Can you work these out from the model? Positions are in its coordinate system, mm. A direction names the side the tool comes from. Round coordinates to 2 decimals unless told otherwise and drop trailing zeros. Write each loop counter-clockwise with the first axis right and the second up, starting at its lowest first coordinate (ties: lowest second). Pieces come first, ordered by that corner, then holes. Notation, with made-up numbers: (35, 60.5) -> (77, 60.5) arc R26 cw to (77, 74.5) -> close; hole circle Ø6 at (54.5, -40). An arc over 180 degrees is marked (long way). Write item = value, one per line. Start each with the question number.
1) Thinking about a two-plate mould opening in X: for faces 1 (the face through (-56.53, 26.78, 0.99)), 2 (the face through (-45, -47.4, 16)), 3 (the face through (15, -42.9, 1)), which applies, +X half, -X half, draft (parallel to the pull), parting line (faces both ways), or undercut?
2) If I drill on line 1 (Y direction, x = 27.5, z = 15.75); line 2 (X direction, y = -44.5, z = 6.25); line 3 (Z direction, x = -13.5, y = 5.5), over which ranges is the centre line in solid material (lowest first)?
3) Imagine slicing it at B-B, the plane z = 11.5. Please give me the cut outline in (x, y).
4) Imagine slicing it at D-D, the plane z = 4. Please give me the cut outline in (x, y), then the cut area to 3 significant figures.
5) For faces 4 (the face through (-27.068, 3.734, 0.986)), 5 (the face through (-34.01, -42.94, 0.99)), 6 (the face through (26.01, -43.743, 8.902)), which set-ups out of +Z, -Z, +X, -X, +Y, -Y let a thin tool reach every point of the face, with its end or its side?
6) I'm going to push flat-ended pins straight in: pin 1 (5.5 mm diameter, centred on x = 20.53, y = 20.83, fed in from +Z); pin 2 (1.4 mm diameter, centred on x = 28, y = -47, fed in from +Z); pin 3 (0.6 mm diameter, centred on x = -9, z = 1.5, fed in from -Y). Where does each tip first touch, or does it pass through?
7) Imagine slicing it at A-A, the plane y = 9. Please give me the cut outline in (x, z).
8) Imagine slicing it at C-C, the plane x = -22.5. Please give me the cut outline in (y, z), then the cut area to 3 significant figures.
from build123d import *

# Parameters (mm, degrees)
SKETCH1_R           = 13
SKETCH1_R_2         = 3
BOSS_EXTRUDE1_DEPTH = 2
SKETCH2_R           = 3.3
BOSS_EXTRUDE2_DEPTH = 14
SKETCH3_R           = 1.4
CUT_EXTRUDE1_DEPTH  = 10


with BuildPart() as part:
    # Sketch1 → Boss-Extrude1 (new body)
    with BuildSketch(Plane.XY):
        with BuildLine():
            Line((30.587032828, 29.429180606), (-49.522529265, 29.429180606))
            ThreePointArc((-49.522529265, 29.429180606), (-56.615313692, 26.706515756), (-60.064461355, 19.937182317))
            Line((-60.064461355, 19.937182317), (-65.933159759, -35.899753171))
            ThreePointArc((-65.933159759, -35.899753171), (-55.634580371, -52.232565016), (-37.345276376, -46.042020648))
            ThreePointArc((-37.345276376, -46.042020648), (-33.948223744, -42.907324122), (-29.467749897, -41.770819394))
            Line((-29.467749897, -41.770819394), (10.53225346, -41.770819394))
            ThreePointArc((10.53225346, -41.770819394), (15.012727307, -42.907324122), (18.409779939, -46.042020648))
            ThreePointArc((18.409779939, -46.042020648), (36.699083934, -52.232565016), (46.997663323, -35.899753171))
            Line((46.997663323, -35.899753171), (41.128964919, 19.937182317))
            ThreePointArc((41.128964919, 19.937182317), (37.679817255, 26.706515756), (30.587032828, 29.429180606))
        make_face()
        with Locations((-39.467748218, -0.170819394)):
            Circle(SKETCH1_R, mode=Mode.SUBTRACT)
        with Locations(Location((20.532251782, -0.170819394, 0), (0, 0, 180))):
            Circle(SKETCH1_R, mode=Mode.SUBTRACT)
        with Locations((-39.467748218, 20.829180606)):
            Circle(SKETCH1_R_2, mode=Mode.SUBTRACT)
        with Locations(Location((20.532251782, 20.829180606, 0), (0, 0, 180))):
            Circle(SKETCH1_R_2, mode=Mode.SUBTRACT)
    extrude(amount=BOSS_EXTRUDE1_DEPTH)

    # Sketch2 → Boss-Extrude2 (add)
    with BuildSketch(Plane.XY.offset(2)):
        with Locations((-46.467748218, -46.670819394)):
            Circle(SKETCH2_R)
        with Locations(Location((27.532251782, -46.670819394, 0), (0, 0, 180))):
            Circle(SKETCH2_R)
    extrude(amount=BOSS_EXTRUDE2_DEPTH)

    # Sketch3 → Cut-Extrude1 (cut)
    with BuildSketch(Plane.XY.offset(16)):
        with Locations((-46.467748218, -46.670819394)):
            Circle(SKETCH3_R)
        with Locations(Location((27.532251782, -46.670819394, 0), (0, 0, 180))):
            Circle(SKETCH3_R)
    extrude(amount=-CUT_EXTRUDE1_DEPTH, mode=Mode.SUBTRACT)


solid = part.part
Reported:
q1.face_1 = -X half
q1.face_2 = draft
q1.face_3 = undercut
q2.line_1 = -49.97 to -48.07, -45.27 to -43.37
q2.line_2 = -48.95 to -43.98, 25.05 to 30.02
q2.line_3 = 0 to 2
q3.outline = circle Ø6.6 at (-46.47, -46.67); circle Ø6.6 at (27.53, -46.67); hole circle Ø2.8 at (-46.47, -46.67); hole circle Ø2.8 at (27.53, -46.67)
q4.outline = circle Ø6.6 at (-46.47, -46.67); circle Ø6.6 at (27.53, -46.67)
q4.area = 68.4 mm²
q5.face_4 = +Z, -Z
q5.face_5 = +Z, -Z, -Y
q5.face_6 = +Z
q6.pin_1 = through
q6.pin_2 = 6
q6.pin_3 = -41.77
q7.outline = (-61.21, 0) -> (-48.68, 0) -> (-48.68, 2) -> (-61.21, 2) -> close; (-30.25, 0) -> (11.32, 0) -> (11.32, 2) -> (-30.25, 2) -> close; (29.75, 0) -> (42.28, 0) -> (42.28, 2) -> (29.75, 2) -> close
q8.outline = (-41.77, 0) -> (29.43, 0) -> (29.43, 2) -> (-41.77, 2) -> close
q8.area = 142 mm²
